```python
from build123d import *

# Parameters (mm, degrees)
SKETCH2_R           = 6.5
BOSS_EXTRUDE2_DEPTH = 5.5
SKETCH1_R           = 2.6
CUT_EXTRUDE1_DEPTH  = 21.193250236


with BuildPart() as part:
    # Sketch2 → Boss-Extrude2 (new body)
    with BuildSketch(Plane.XY):
        with Locations((7.165538907, 7.311965881)):
            Circle(SKETCH2_R)
    extrude(amount=-BOSS_EXTRUDE2_DEPTH)

    # Sketch1 → Cut-Extrude1 (cut, through all)
    with BuildSketch(Plane.XY):
        with Locations((7.165538907, 7.311965881)):
            Circle(SKETCH1_R)
        with BuildLine():
            Line((10.969559419, 10.723771247), (10.969559419, 13.011721187))
            add(Edge.make_bspline(
                [(10.969559419, 13.011721187), (10.958646548, 13.475622363), (10.162270372, 13.509138157), (10.169559419, 13.215491328)],
                knots=[0, 0, 0, 0, 1, 1, 1, 1], degree=3))
            Line((10.169559419, 13.215491328), (10.169559419, 10.721114654))
            add(Edge.make_bspline(
                [(10.169559419, 10.721114654), (10.169559419, 10.211921076), (10.969559419, 10.170868336), (10.969559419, 10.723771247)],
                knots=[0, 0, 0, 0, 1, 1, 1, 1], degree=3))
        make_face()
        with BuildLine():
            Line((13.069064354, 4.307945368), (10.57468768, 4.307945368))
            add(Edge.make_bspline(
                [(10.57468768, 4.307945368), (10.065494102, 4.307945368), (10.024441362, 3.507945368), (10.577344274, 3.507945368)],
                knots=[0, 0, 0, 0, 1, 1, 1, 1], degree=3))
            Line((10.577344274, 3.507945368), (12.865294213, 3.507945368))
            add(Edge.make_bspline(
                [(12.865294213, 3.507945368), (13.329195389, 3.518858239), (13.362711183, 4.315234416), (13.069064354, 4.307945368)],
                knots=[0, 0, 0, 0, 1, 1, 1, 1], degree=3))
        make_face()
        with BuildLine():
            Line((4.161518395, 1.408440433), (4.161518395, 3.902817107))
            add(Edge.make_bspline(
                [(4.161518395, 3.902817107), (4.161518395, 4.412010686), (3.361518395, 4.453063426), (3.361518395, 3.900160514)],
                knots=[0, 0, 0, 0, 1, 1, 1, 1], degree=3))
            Line((3.361518395, 3.900160514), (3.361518395, 1.612210574))
            add(Edge.make_bspline(
                [(3.361518395, 1.612210574), (3.372431266, 1.148309399), (4.168807442, 1.114793605), (4.161518395, 1.408440433)],
                knots=[0, 0, 0, 0, 1, 1, 1, 1], degree=3))
        make_face()
        with BuildLine():
            Line((1.26201346, 10.315986393), (3.756390133, 10.315986393))
            add(Edge.make_bspline(
                [(3.756390133, 10.315986393), (4.265583712, 10.315986393), (4.306636452, 11.115986393), (3.75373354, 11.115986393)],
                knots=[0, 0, 0, 0, 1, 1, 1, 1], degree=3))
            Line((3.75373354, 11.115986393), (1.465783601, 11.115986393))
            add(Edge.make_bspline(
                [(1.465783601, 11.115986393), (1.001882425, 11.105073522), (0.968366631, 10.308697346), (1.26201346, 10.315986393)],
                knots=[0, 0, 0, 0, 1, 1, 1, 1], degree=3))
        make_face()
    extrude(amount=-CUT_EXTRUDE1_DEPTH, mode=Mode.SUBTRACT)


solid = part.part
```
Work out the finished part from the listing and answer in its coordinate system (mm). A direction names the side the tool comes from. Give positions to 0.01 mm unless a question says otherwise; leave off trailing zeros. Loops run counter-clockwise (first coordinate to the right, second up) from the corner with the lowest first, then second, coordinate; pieces in that order, holes last. Notation, with made-up numbers: (54, 18.5) -> (68, 18.5) arc R20 cw to (68, 31.5) -> close; hole circle Ø10 at (80, 45). An arc over 180 degrees is marked (long way). Put each result on its own line as item: value. Start each with the question number.
Item 1: Which of the six approach directions +Z, -Z, +X, -X, +Y, -Y give full straight-line access (tool end or side, diameter ignored) to faces 1 (the face through (11, 3.508, -3)), 2 (the face through (10, 7, 0)), 3 (the face through (3, 11.116, -3)), 4 (the face through (10.17, 12, -3)), 5 (the face through (3.362, 3, -3))?
Item 2: The part is cut by section A-A (x = 8). Give the vertices of the cut face in (y, z).
Item 3: The part is cut by section B-B (y = 11.75). Give the vertices of the cut face in (x, z), then the cut area to 3 significant figures.
Item 4: The mould has two halves that part along Y. Classify faces 6 (the face through (0.826, 5.877, -2.712)), 7 (the face through (3, 10.316, -3)), 8 (the face through (12, 4.308, -3)), 9 (the face through (5.73, 13.65, -2.71)): released by +Y, released by -Y, zero draft, split by the parting line, or undercut.
Item 5: The part is cut by section C-C (y = 4.5). Give the vertices of the cut face in (x, z).
Item 6: Find the intervals of material crossed by L1, parallel to X at y = 2.5, z = -3.9; L2, parallel to X at y = 5.5, z = -4.6; L3, parallel to Y at x = 3, z = -3.35, in increasing order. Write a range as [from, to].
Item 7: Each of these flat-tipped pins is pushed along its axis until it touches: P1, Ø2, axis at x = 4.5, z = -1.5, coming from the +Y side; P2, Ø0.9, axis at y = 12, z = -3.5, coming from the -X side; P3, Ø0.6, axis at x = 11.5, z = -4, coming from the +Y side. Where does it stop, or does it pass through?
Answers below:
1. face 1: +Z, -Z, +X
1. face 2: +Z, +X, -X, +Y, -Y
1. face 3: +Z, -Z, -X
1. face 4: +Z, -Z, +Y
1. face 5: +Z, -Z, -Y
2. outline: (0.87, -5.5) -> (4.85, -5.5) -> (4.85, 0) -> (0.87, 0) -> close; (9.77, -5.5) -> (13.76, -5.5) -> (13.76, 0) -> (9.77, 0) -> close
3. outline: (2.42, -5.5) -> (10.17, -5.5) -> (10.17, 0) -> (2.42, 0) -> close; (10.97, -5.5) -> (11.91, -5.5) -> (11.91, 0) -> (10.97, 0) -> close
3. area: 47.8 mm2
4. face 6: split by the parting line
4. face 7: undercut
4. face 8: undercut
4. face 9: released by +Y
5. outline: (1.31, -5.5) -> (13.03, -5.5) -> (13.03, 0) -> (1.31, 0) -> close
6. L1: [2.8, 3.36], [4.16, 11.54]
6. L2: [0.92, 5.3], [9.03, 13.41]
6. L3: [2.32, 10.32], [11.12, 12.3]
7. P1: y = 13.59
7. P2: x = 2.24
7. P3: y = 12.41
